from build123d import *

# Parameters (mm, degrees)
F0_R      = 12.5
F1_DEPTH  = 27
F2_R      = 12.25
F3_DEPTH  = 30.8
F4_R      = 3.5
F5_DEPTH  = 2.5
F6_R      = 2
F7_DEPTH  = 9.5
F9_DEPTH  = 8
F10_R     = 1.5
F11_DEPTH = 6
F12_R     = 4
F13_DEPTH = 2
F14_R     = 11.5
F15_DEPTH = 2
F16_R     = 1
F17_DEPTH = 3
F18_R     = 7
F19_DEPTH = 4
F20_W     = 16
F20_H     = 5
F21_DEPTH = 2.5


with BuildPart() as f1:
    # F0 (on Front) → F1 (new body)
    with BuildSketch(Plane.XZ):
        Circle(F0_R)
    extrude(amount=F1_DEPTH)

    # F2 (on face) → F3 (join)
    with BuildSketch(Plane.XZ.offset(27)):
        Circle(F2_R)
    extrude(amount=F3_DEPTH)

    # F4 (on face) → F5 (join)
    with BuildSketch(Plane(origin=(0, 0, 0), x_dir=(-1, 0, 0), z_dir=(0, 1, 0))):
        Circle(F4_R)
    extrude(amount=F5_DEPTH)

    # F6 (on face) → F7 (join)
    with BuildSketch(Plane(origin=(0, 2.5, 0), x_dir=(-1, 0, 0), z_dir=(0, 1, 0))):
        Circle(F6_R)
    extrude(amount=F7_DEPTH)

    # F8 (on face) → F9 (cut)
    with BuildSketch(Plane(origin=(0, 12, 0), x_dir=(-1, 0, 0), z_dir=(0, 1, 0))):
        with BuildLine():
            ThreePointArc((1.322876, 1.5), (0, 2), (-1.322876, 1.5))
            Line((-1.322876, 1.5), (1.322876, 1.5))
        make_face()
    extrude(amount=-F9_DEPTH, mode=Mode.SUBTRACT)

    # F10 (on face) → F11 (cut)
    with BuildSketch(Plane(origin=(0, 0, 0), x_dir=(-1, 0, 0), z_dir=(0, 1, 0))):
        with Locations((8.5, 0)):
            Circle(F10_R)
        with Locations((-8.5, 0)):
            Circle(F10_R)
    extrude(amount=-F11_DEPTH, mode=Mode.SUBTRACT)

    # F12 (on face) → F13 (join)
    with BuildSketch(Plane.XZ.offset(57.8)):
        Circle(F12_R)
    extrude(amount=F13_DEPTH)

    # F14 (on face) → F15 (join)
    with BuildSketch(Plane.XZ.offset(59.8)):
        Circle(F14_R)
    extrude(amount=F15_DEPTH)

    # F16 (on face) → F17 (join)
    with BuildSketch(Plane.XZ.offset(61.8)):
        Circle(F16_R)
    extrude(amount=F17_DEPTH)

    # F18 (on face) → F19 (join)
    with BuildSketch(Plane.XZ.offset(64.8)):
        Circle(F18_R)
    extrude(amount=F19_DEPTH)

    # F20 (on face) → F21 (join)
    with BuildSketch(Plane.XZ.offset(61.8)):
        with Locations((0, -6.5)):
            Rectangle(F20_W, F20_H)
    extrude(amount=F21_DEPTH)


solid = f1.part
Read the model definition and answer for the solid it produces. Units are mm, in the model's axes. A direction names the side the tool comes from. Coordinates: 2 decimals unless noted, no trailing zeros. Order: outer loops, then holes, each group sorted by start corner. A loop starts at its lowest first (then second) coordinate and runs counter-clockwise, first axis right, second up. Notation, with made-up numbers: M -38.75,46 L -20.75,46 A13 ccw -20.75,59 Z; hole C -9,44.25 d9. An arc over 180 degrees is marked long. Put each result on its own line as item: value. Start each with the question number.
Item 1: Section B-B, the plane y = -45 is taken. Determine the outline of the cut face in (x, z).
Item 2: The mould has two halves that part along X. Classify faces 1 (the face through (8, -63, -7)), 2 (the face through (0, -68.8, 0)), 3 (the face through (9, -6, 0)): +X half, -X half, draft (parallel to the pull), parting line (faces both ways), or undercut.
Item 3: Section A-A, the plane z = 5 is taken. Determine the outline of the cut face in (x, y), plus the area to 3 significant figures.
Item 4: Given pin 1 Ø6 at (y, z) = (-10, -7) entering from +X; pin 2 Ø3 at (x, z) = (-4.5, -9) entering from +Y; pin 3 Ø4 at (x, z) = (-8.5, -8) entering from -Y, each flat-ended and moving along its own axis, determine where each tip first touches the part or whether it passes through.
Item 5: For faces 4 (the face through (0, -61.8, -10)), 5 (the face through (0, -63, -1)), 6 (the face through (11.923, -13.311, 3.755)), 7 (the face through (-8, -63, -7)), 8 (the face through (10, -3, 0)), determine the directions among +Z, -Z, +X, -X, +Y, -Y from which every point of the face is accessible in a straight line to the end or side of a thin tool.
Item 6: Section C-C, the plane y = -9 is taken. Determine the outline of the cut face in (x, z).
Item 7: Consider probe 1 along Y at (x, z) = (1, 5.25); probe 2 along Y at (x, z) = (5.5, 8.25); probe 3 along Y at (x, z) = (0.75, -1). Determine where each line is inside the solid, lowest interval first. Write a range as [from, to].
Computed:
1. outline: C 0,0 d24.5
2. face 1: +X half
2. face 2: draft
2. face 3: undercut
3. outline: M -11.46,-27 L -11.18,-27 L -11.18,-57.8 L 11.18,-57.8 L 11.18,-27 L 11.46,-27 L 11.46,0 L -11.46,0 Z; M -10.36,-61.8 L 10.36,-61.8 L 10.36,-59.8 L -10.36,-59.8 Z; M -4.9,-68.8 L 4.9,-68.8 L 4.9,-64.8 L -4.9,-64.8 Z
3. area: 1,390 mm2
4. pin 1: stops at x = 11.84
4. pin 2: stops at y = 0
4. pin 3: stops at y = -64.3
5. face 4: -Z, +X, -X, -Y
5. face 5: none
5. face 6: +Y, -Y
5. face 7: +Z, -Z, -X, -Y
5. face 8: +Y
6. outline: C 0,0 d25
7. probe 1: y = [-68.8, -64.8], [-61.8, -59.8], [-57.8, 0]
7. probe 2: y = [-61.8, -59.8], [-57.8, 0]
7. probe 3: y = [-68.8, -64.8], [-61.8, 12]
